Autodesk Inventor part; units mm, degrees
ref_plane "YZ Plane" through (0, 0, 0) normal (1, 0, 0) x (0, 1, 0)
ref_plane "XZ Plane" through (0, 0, 0) normal (0, 1, 0) x (-1, 0, 0)
ref_plane "XY Plane" through (0, 0, 0) normal (0, 0, 1) x (1, 0, 0)
sketch "Sketch1" plane through (0, 0, 0) normal (0, 0, 1) x (1, 0, 0)
  line L0 (-37.6, 3.81) -> (-12.2, 3.81)
  line L1 (-12.2, 3.81) -> (-12.2, -3.81)
  line L2 (-12.2, -3.81) -> (-37.6, -3.81)
  line L3 (-37.6, -3.81) -> (-37.6, 3.81)
  line L4 (-52.64, 0) -> (52.64, 0)
  line L5 (0, -32.0572) -> (0, 10.9036)
  line L6 (12.2, 3.81) -> (37.6, 3.81)
  line L7 (37.6, 3.81) -> (37.6, -3.81)
  line L8 (37.6, -3.81) -> (12.2, -3.81)
  line L9 (12.2, -3.81) -> (12.2, 3.81)
  line L10 (-9.3568, 0) -> (3.5049, 0)
  arc A0 (-12.2, -3.81) -> (12.2, -3.81) centre (0, -6.6323) ccw
  arc A1 (-19.08, -3.81) -> (19.08, -3.81) centre (0, -6.6323) ccw
  point P0 (0, 0)
  dimension "d0" = 7.62
  dimension "d2" = 7.62
  dimension "d19" = 25.4
  dimension "d20" = 25.4
  dimension "d31" = 24.4
  dimension "d32" = 12.5222
extrude "Extrusion3" add sketch "Sketch1" along normal blind 26 contours L0 L1 L4 L3 | L4 L1 L2 L3 | L9 L4 L7 L8 | L9 L6 L7 L4
extrude "Extrusion6" add sketch "Sketch1" along normal blind 26 contours A0 L5 A1 L2 | A0 L8 A1 L5
sketch "Sketch5" plane through (-37.6, 3.81, 0) normal (0, 1, 0) x (1, 0, 0)
  circle A0 centre (7.9375, -12.7) radius 1.5875
  circle A1 centre (66.675, -12.7) radius 1.5875
  point P0 (37.6, 0)
extrude "Extrusion8" cut sketch "Sketch5" against normal blind 10.16
sketch "Sketch6" plane through (0, 0, 0) normal (0, 0, -1) x (-1, 0, 0)
  circle A0 centre (0.0788, -7.3494) radius 12.1158
  dimension "d33" = 24.2316
fillet "Fillet4" radius 3.175 2 edges at (-19.08, -3.81, 13) (19.08, -3.81, 13)
equation "\"d2\" = d0"
properties part number "motor mounts"
Verification items for the finished model (mm, model axes). A direction names the side the tool comes from. Give positions to 0.01 mm unless a question says otherwise; leave off trailing zeros. Order: outer loops, then holes, each group sorted by start corner. A loop starts at its lowest first (then second) coordinate and runs counter-clockwise, first axis right, second up. Notation, with made-up numbers: M -37.75,28 L -9.75,28 A13 cw -9.75,50 Z; hole C 47.25,75.5 d3. An arc over 180 degrees is marked long. Answer as a JSON object with one key per item and string values. Group by question number.
1) Depth check by flat-ended pin: pin 1 Ø12 at (x, z) = (-9, 4) entering from -Y; pin 2 Ø4 at (y, z) = (-14, 11.5) entering from -X; pin 3 Ø5 at (y, z) = (-9.5, 17) entering from -X. Enter the tip coordinate at first touch or a pass-through.
2) Cross-section at C-C (y = -13.75). Enter the section's corners in (x, z), then the cut area to 3 significant figures.
3) Scan lines: line 1 along X through (y, z) = (-3.5, 6.5); line 2 along X through (y, z) = (-7, 6); line 3 along Y through (x, z) = (0, 20.5). Record each from-to range of solid material in increasing order. Write a range as [from, to].
4) Mould release check, pull along Z, two halves, no side actions. Record for faces 1 (the face through (-6, -19, 0)), 2 (the face through (-25, 3.81, 13)), 3 (the face through (27.49, 0.05, 12.63)): released by +Z, released by -Z, zero draft, split by the parting line, or undercut.
5) Access from +Z, -Z, +X, -X, +Y, -Y to the whole of each face (thin tool, end or side, straight path). Record for faces 4 (the face through (-32, -3.81, 13)), 5 (the face through (12.2, 0, 13)), 6 (the face through (37.6, 0, 13)), 7 (the face through (32, -3.81, 13)).
6) Cross-section at D-D (x = 28.5). Enter the section's corners in (y, z), then the cut area to 3 significant figures.
7) Cross-section at A-A (z = 12.7). Give the number of separate pieces and of enclosed holes in the cut face, then the cut area to 3 significant figures.
8) Cross-section at B-B (y = -2.5). Enter the section's corners in (x, z) (1 decimal).
Result sheet:
{
 "1": {"pin 1": "stops at y = -25.69", "pin 2": "stops at x = -18.53", "pin 3": "stops at x = -19.28"},
 "2": {"outline": "M -17.93,0 L -10.3,0 L -10.3,26 L -17.93,26 Z; M 10.3,0 L 17.93,0 L 17.93,26 L 10.3,26 Z", "area": "396 mm2"},
 "3": {"line 1": "x = [-37.6, -12.2], [12.2, 37.6]", "line 2": "x = [-19.28, -12.52], [12.52, 19.28]", "line 3": "y = [-25.92, -19.15]"},
 "4": {"face 1": "released by -Z", "face 2": "zero draft", "face 3": "undercut"},
 "5": {"face 4": "+Z, -Z, -X, -Y", "face 5": "+Z, -Z, +Y", "face 6": "+Z, -Z, +X, +Y, -Y", "face 7": "+Z, -Z, +X, -Y"},
 "6": {"outline": "M -3.81,0 L 3.81,0 L 3.81,11.22 L -3.81,11.22 Z; M -3.81,14.18 L 3.81,14.18 L 3.81,26 L -3.81,26 Z", "area": "176 mm2"},
 "7": {"separate pieces": "3", "enclosed holes": "0", "area": "720 mm2"},
 "8": {"outline": "M -37.6,0 L -12.2,0 L -12.2,26 L -37.6,26 Z; M 12.2,0 L 37.6,0 L 37.6,26 L 12.2,26 Z; hole C -29.7,12.7 d3.2; hole C 29.1,12.7 d3.2"}
}
